from build123d import *

# Parameters (mm, degrees)
SKETCH1_R                    = 18.4
BOSS_EXTRUDE1_DEPTH          = 24.3
SKETCH2_R                    = 17.4
BOSS_EXTRUDE2_DEPTH          = 30
SKETCH3_R                    = 6
BOSS_EXTRUDE3_DEPTH          = 6.5
FILLET1_R                    = 0.5
SKETCH4_R                    = 3
BOSS_EXTRUDE4_DEPTH          = 15
CUT_EXTRUDE1_START           = -12
CUT_EXTRUDE1_DEPTH           = 12
F_3_0_3_DIAMETER_HOLE1_D     = 3
F_3_0_3_DIAMETER_HOLE1_DEPTH = 3
F_3_0_3_DIAMETER_HOLE1_TIP   = 0.901290929
CUT_EXTRUDE2_DEPTH           = 1
SKETCH9_R                    = 4
BOSS_EXTRUDE5_DEPTH          = 1
FILLET2_R                    = 0.5
SKETCH10_R                   = 14
BOSS_EXTRUDE6_DEPTH          = 1.5
SKETCH11_W                   = 3.5
SKETCH11_H                   = 1
BOSS_EXTRUDE7_DEPTH          = 5.6
FILLET3_R                    = 0.5
SKETCH13_R                   = 9
BOSS_EXTRUDE8_DEPTH          = 3
SKETCH14_R                   = 1.5
BOSS_EXTRUDE9_DEPTH          = 8.55
FILLET4_R                    = 0.5
SKETCH15_W                   = 3
SKETCH15_H                   = 16.7
SKETCH16_R                   = 14
BOSS_EXTRUDE10_DEPTH         = 1
CUT_EXTRUDE3_START           = 12
SKETCH17_W                   = 3.5
SKETCH17_H                   = 13
CUT_EXTRUDE3_DEPTH           = 42.460359146


with BuildPart() as part:
    # Sketch1 → Boss-Extrude1 (new body)
    with BuildSketch(Plane.XY):
        Circle(SKETCH1_R)
    extrude(amount=BOSS_EXTRUDE1_DEPTH)

    # Sketch2 → Boss-Extrude2 (add)
    with BuildSketch(Plane(origin=(0, 0, 0), x_dir=(-1, 0, 0), z_dir=(0, 0, -1))):
        with Locations(Location((0, 0, 0), (0, 0, 180))):
            Circle(SKETCH2_R)
    extrude(amount=BOSS_EXTRUDE2_DEPTH)

    # Sketch3 → Boss-Extrude3 (add)
    with BuildSketch(Plane.XY.offset(24.3)):
        with Locations(Location((7, 0, 0), (0, 0, 180))):
            Circle(SKETCH3_R)
    extrude(amount=BOSS_EXTRUDE3_DEPTH)

    # Fillet1
    fillet1_edges = [part.edges().sort_by_distance(p)[0] for p in [
        (13, 0, 30.8),
    ]]
    fillet(fillet1_edges, radius=FILLET1_R)

    # Sketch4 → Boss-Extrude4 (add)
    with BuildSketch(Plane.XY.offset(30.8)):
        with Locations((7, 0)):
            Circle(SKETCH4_R)
    extrude(amount=BOSS_EXTRUDE4_DEPTH)

    # Sketch5 → Cut-Extrude1 (cut)
    with BuildSketch(Plane.XY.offset(45.8).offset(CUT_EXTRUDE1_START)):
        with BuildLine():
            Line((5.503337045, 2.6), (8.496662955, 2.6))
            ThreePointArc((8.496662955, 2.6), (7, 3), (5.503337045, 2.6))
        make_face()
    extrude(amount=CUT_EXTRUDE1_DEPTH, mode=Mode.SUBTRACT)

    # Ø3.0 (3) Diameter Hole1
    with Locations(Plane.XY.offset(24.3)):
        with Locations((-13.423393759, 7.75), (-13.423393759, -7.75), (0, -15.5), (13.423393759, 7.75), (0, 15.5), (13.423393759, -7.75)):
            Hole(F_3_0_3_DIAMETER_HOLE1_D / 2, depth=F_3_0_3_DIAMETER_HOLE1_DEPTH)
            with Locations((0, 0, -(F_3_0_3_DIAMETER_HOLE1_DEPTH + F_3_0_3_DIAMETER_HOLE1_TIP / 2))):  # 118° drill point
                Cone(0, F_3_0_3_DIAMETER_HOLE1_D / 2, F_3_0_3_DIAMETER_HOLE1_TIP, mode=Mode.SUBTRACT)

    # Sketch8 → Cut-Extrude2 (cut)
    with BuildSketch(Plane.XY.offset(24.3)):
        with BuildLine():
            ThreePointArc((10.116155685, 7.342574083), (-12.5, 0), (10.116155685, -7.342574083))
            ThreePointArc((10.116155685, -7.342574083), (-1.05978604, 0), (10.116155685, 7.342574083))
        make_face()
    extrude(amount=-CUT_EXTRUDE2_DEPTH, mode=Mode.SUBTRACT)

    # Sketch9 → Boss-Extrude5 (add)
    with BuildSketch(Plane(origin=(0, 0, -30), x_dir=(-1, 0, 0), z_dir=(0, 0, -1))):
        Circle(SKETCH9_R)
    extrude(amount=BOSS_EXTRUDE5_DEPTH)

    # Fillet2
    fillet2_edges = [part.edges().sort_by_distance(p)[0] for p in [
        (4, 0, -31),
    ]]
    fillet(fillet2_edges, radius=FILLET2_R)

    # Sketch11 → Boss-Extrude7 (add)
    with BuildSketch(Plane(origin=(0, 0, -30), x_dir=(-1, 0, 0), z_dir=(0, 0, -1))):
        with Locations((0, 12.05)):
            Rectangle(SKETCH11_W, SKETCH11_H)
        with Locations((0, -12.05)):
            Rectangle(SKETCH11_W, SKETCH11_H)
    extrude(amount=BOSS_EXTRUDE7_DEPTH)

    # Fillet3
    fillet3_edges = [part.edges().sort_by_distance(p)[0] for p in [
        (1.75, 12.05, -35.6),
        (-1.75, 12.05, -35.6),
        (-1.75, -12.05, -35.6),
        (1.75, -12.05, -35.6),
    ]]
    fillet(fillet3_edges, radius=FILLET3_R)

    # Sketch14 → Boss-Extrude9 (add)
    with BuildSketch(Plane(origin=(0, 0, -31), x_dir=(-1, 0, 0), z_dir=(0, 0, -1))):
        Circle(SKETCH14_R)
    extrude(amount=BOSS_EXTRUDE9_DEPTH)

    # Fillet4
    # the kernel refuses this fillet: 0.5 mm, written as the material it takes off along each edge
    with BuildSketch(Plane(origin=(7, 0, 45.8), x_dir=(0.4622655728594592, 0.8867415295050277, 0), z_dir=(0.8867415295050277, -0.4622655728594592, 0))) as fillet4_piece_1:
        with BuildLine():
            CenterArc((3 - FILLET4_R, -FILLET4_R), FILLET4_R, 0, 90)
            Line((3 - FILLET4_R, 0), (3 - FILLET4_R, FILLET4_R * 0.02))
            Line((3 - FILLET4_R, FILLET4_R * 0.02), (3 + FILLET4_R * 0.02, FILLET4_R * 0.02))
            Line((3 + FILLET4_R * 0.02, FILLET4_R * 0.02), (3 + FILLET4_R * 0.02, -FILLET4_R))
            Line((3 + FILLET4_R * 0.02, -FILLET4_R), (3, -FILLET4_R))
        make_face()
    revolve(axis=Axis((7, 0, 45.8), (0, 0, 1)), revolution_arc=297.533397677, mode=Mode.SUBTRACT)
    with BuildSketch(Plane(origin=(7, 0, 45.8), x_dir=(1, 0, 0), z_dir=(0, -1, 0))) as fillet4_piece_2:
        with BuildLine():
            CenterArc((3 - FILLET4_R, -FILLET4_R), FILLET4_R, 0, 90)
            Line((3 - FILLET4_R, 0), (3 - FILLET4_R, FILLET4_R * 0.02))
            Line((3 - FILLET4_R, FILLET4_R * 0.02), (3 + FILLET4_R * 0.02, FILLET4_R * 0.02))
            Line((3 + FILLET4_R * 0.02, FILLET4_R * 0.02), (3 + FILLET4_R * 0.02, -FILLET4_R))
            Line((3 + FILLET4_R * 0.02, -FILLET4_R), (3, -FILLET4_R))
        make_face()
    revolve(axis=Axis((7, 0, 45.8), (0, 0, 1)), revolution_arc=117.379597562, mode=Mode.SUBTRACT)


with BuildPart() as body_2:
    # Sketch10 → Boss-Extrude6 (new body)
    with BuildSketch(Plane(origin=(0, 0, -33), x_dir=(-1, 0, 0), z_dir=(0, 0, -1))):
        Circle(SKETCH10_R)
    extrude(amount=BOSS_EXTRUDE6_DEPTH)


    add(part.part)  # Revolve1 merges part


with BuildPart() as body_3:
    # Sketch13 → Boss-Extrude8 (new body)
    with BuildSketch(Plane(origin=(0, 0, -36.5), x_dir=(-1, 0, 0), z_dir=(0, 0, -1))):
        Circle(SKETCH13_R)
    extrude(amount=BOSS_EXTRUDE8_DEPTH)


with BuildPart() as body_2_1:
    add(body_2.part)

    add(body_3.part)  # Revolve1 merges body 3
    # Sketch15 → Revolve1 (revolve)
    with BuildSketch(Plane(origin=(0, 0, 0), x_dir=(1, 0, 0), z_dir=(0, 1, 0))):
        with Locations((-15.5, 38.35)):
            Rectangle(SKETCH15_W, SKETCH15_H)
    revolve(axis=Axis((0, 0, -30), (0, 0, 1)))

    # Sketch16 → Boss-Extrude10 (add)
    with BuildSketch(Plane(origin=(0, 0, -46.7), x_dir=(-1, 0, 0), z_dir=(0, 0, -1))):
        Circle(SKETCH16_R)
    extrude(amount=-BOSS_EXTRUDE10_DEPTH)

    # Sketch17 → Cut-Extrude3 (cut, through all)
    with BuildSketch(Plane(origin=(0, 0, 0), x_dir=(0, 0, -1), z_dir=(1, 0, 0)).offset(CUT_EXTRUDE3_START)):
        with Locations((34.75, 0)):
            Rectangle(SKETCH17_W, SKETCH17_H)
    extrude(amount=CUT_EXTRUDE3_DEPTH, mode=Mode.SUBTRACT)


solid = body_2_1.part
Could you check a few things on this model? Use its own coordinates, in mm. A direction names the side the tool comes from. Coordinates: 2 decimals unless noted, no trailing zeros. Order: outer loops, then holes, each group sorted by start corner. A loop starts at its lowest first (then second) coordinate and runs counter-clockwise, first axis right, second up. Notation, with made-up numbers: (59, -3.5) - (94, -3.5) arc R17 ccw to (94, 24.5) - close; hole circle Ø3 at (16.5, -20). An arc over 180 degrees is marked (long way). Answer in a Markdown table with one row per item. Add a question column.
(1) If we section it at C-C, the plane x = 7: State how many separate pieces and enclosed holes the cut face has, then the cut area to 3 significant figures.
(2) If we section it at D-D, the plane z = 28.5: Please give me the cut outline in (x, y), then the cut area to 3 significant figures.
(3) If we section it at B-B, the plane z = 19: Please give me the cut outline in (x, y).
(4) If we mould it in two halves opening along X, with no side actions, what happens to faces 1 (the face through (15.4, 7.7, -30)), 2 (the face through (0.12, 15.269, 20.555)), 3 (the face through (8.384, -2.662, 37.948))? For each: released by +X, released by -X, zero draft, split by the parting line, or undercut.
(5) Will these pins go through, and if not, where does the flat tip stop? pin 1 (1.5 mm diameter, centred on x = 1, z = -31, fed in from +Y); pin 2 (0.5 mm diameter, centred on y = 12, z = -35, fed in from +X); pin 3 (3.5 mm diameter, centred on x = -0.5, z = -31, fed in from -Y); pin 4 (5 mm diameter, centred on y = -7, z = 35.5, fed in from -X).
(6) If we section it at A-A, the plane x = -5: Please give me the cut outline in (y, z).
(7) I need wall thicknesses on L1, parallel to Z at x = 5, y = 5; L2, parallel to Z at x = -7, y = -11; L3, parallel to Y at x = 0, z = 22. Which ranges of each line are inside material? Lowest first, please.
(8) On a 3-axis mill with a long thin cutter (end or side, diameter ignored), from which of +Z, -Z, +X, -X, +Y, -Y can I reach the whole of each face in a straight line? I mean faces 4 (the face through (1.5, 0.07, -31.99)), 5 (the face through (14, 6.5, -35)), 6 (the face through (1.11, 16.51, 22.78)), 7 (the face through (-16.215, -5.106, -38.467)). Say none if no direction works.
Results are:
| question | item | result |
|---|---|---|
| 1 | separate pieces | 2 |
| 1 | enclosed holes | 2 |
| 1 | area | 2,150 mm2 |
| 2 | outline | circle Ø12 at (7, 0) |
| 2 | area | 113 mm2 |
| 3 | outline | circle Ø36.8 at (0, 0) |
| 4 | face 1 | zero draft |
| 4 | face 2 | undercut |
| 4 | face 3 | split by the parting line |
| 5 | pin 1 | stops at y = 17 |
| 5 | pin 2 | stops at x = 12.29 |
| 5 | pin 3 | stops at y = -17.4 |
| 5 | pin 4 | passes through |
| 6 | outline | (-17.71, 0) - (-16.67, 0) - (-16.67, -30) - (-16.25, -30) - (-16.25, -46.7) - (16.25, -46.7) - (16.25, -30) - (16.67, -30) - (16.67, 0) - (17.71, 0) - (17.71, 24.3) - (11.46, 24.3) - (11.46, 23.3) - (-11.46, 23.3) - (-11.46, 24.3) - (-17.71, 24.3) - close; (-7.48, -39.5) - (7.48, -39.5) - (7.48, -36.5) - (-7.48, -36.5) - close; hole (-13.08, -45.7) - (13.08, -45.7) - (13.08, -34.5) - (-13.08, -34.5) - close; hole (-13.08, -33) - (13.08, -33) - (13.08, -30) - (-13.08, -30) - close |
| 7 | L1 | z = -46.7 to -45.7, -39.5 to -36.5, -34.5 to -33, -30 to 30.8 |
| 7 | L2 | z = -46.7 to -45.7, -34.5 to -33, -30 to 24.3 |
| 7 | L3 | y = -18.4 to -17, -14 to 14, 17 to 18.4 |
| 8 | face 4 | none |
| 8 | face 5 | +X |
| 8 | face 6 | +Z |
| 8 | face 7 | -Z |
